Can you work these out from the model? Positions are in its coordinate system, mm. A direction names the side the tool comes from. Round coordinates to 2 decimals unless told otherwise and drop trailing zeros. Loops run counter-clockwise (first coordinate to the right, second up) from the corner with the lowest first, then second, coordinate; pieces in that order, holes last. Notation, with made-up numbers: M -26.75,38 L 13.25,38 A26 cw 13.25,69 Z; hole C 4.5,-30.5 d10. An arc over 180 degrees is marked long. Return JSON: item names as keys, results as strings.
```python
from build123d import *

# Parameters (mm, degrees)
SKETCH_2_W          = 60
SKETCH_2_H          = 39
EXTRUDE_1_DEPTH     = 70
SKETCH_3_R          = 50
EXTRUDE_2_DEPTH     = 43
FILLET_1_R          = 5
FILLET_2_R          = 5
SKETCH_4_R          = 1.5
CUT_EXTRUDE_1_DEPTH = 3.5
SKETCH_5_R          = 1.5
CUT_EXTRUDE_2_DEPTH = 3.5


with BuildPart() as part:
    # 草图2 → 凸台-拉伸1 (new body)
    with BuildSketch(Plane(origin=(0, 0, 0), x_dir=(0, 0, -1), z_dir=(1, 0, 0))):
        Rectangle(SKETCH_2_W, SKETCH_2_H)
    extrude(amount=EXTRUDE_1_DEPTH)

    # 草图3 → 凸台-拉伸2 (add)
    with BuildSketch(Plane(origin=(70, 0, 0), x_dir=(0, 0, -1), z_dir=(1, 0, 0))):
        Circle(SKETCH_3_R)
    extrude(amount=-EXTRUDE_2_DEPTH)

    # 圆角1
    fillet_1_edges = [part.edges().sort_by_distance(p)[0] for p in [
        (70, 0, 50),
    ]]
    fillet(fillet_1_edges, radius=FILLET_1_R)

    # 圆角2
    fillet_2_edges = [part.edges().sort_by_distance(p)[0] for p in [
        (27, 0, 50),
    ]]
    fillet(fillet_2_edges, radius=FILLET_2_R)

    # 草图4 → 切除-拉伸1 (cut)
    with BuildSketch(Plane(origin=(0, 19.5, 0), x_dir=(1, 0, 0), z_dir=(0, 1, 0))):
        with Locations(Location((13, 0, 0), (0, 0, 270))):
            Circle(SKETCH_4_R)
    extrude(amount=-CUT_EXTRUDE_1_DEPTH, mode=Mode.SUBTRACT)

    # 草图5 → 切除-拉伸2 (cut)
    with BuildSketch(Plane.XZ.offset(19.5)):
        with Locations(Location((8, 13.5, 0), (0, 0, 270))):
            Circle(SKETCH_5_R)
        with Locations(Location((8, -13.25, 0), (0, 0, 270))):
            Circle(SKETCH_5_R)
    extrude(amount=-CUT_EXTRUDE_2_DEPTH, mode=Mode.SUBTRACT)


solid = part.part
```
Q1. I'm going to push flat-ended pins straight in: pin 1 Ø12 at (x, y) = (43, 26) entering from -Z; pin 2 Ø3 at (x, y) = (40, 4) entering from +Z; pin 3 Ø1 at (x, y) = (33.5, 25.5) entering from -Z. Where does each tip first touch, or does it pass through?
Results:
{"pin 1": "stops at z = -45.83", "pin 2": "stops at z = 49.94", "pin 3": "stops at z = -43.3"}
Q2. If I drill on line 1 along X through (y, z) = (18.35, 0); line 2 along X through (y, z) = (-18.25, 13.5); line 3 along X through (y, z) = (37, 0.5), over which ranges is the centre line in solid material (lowest first)?
Results:
{"line 1": "x = 0 to 11.5, 14.5 to 70", "line 2": "x = 0 to 6.5, 9.5 to 70", "line 3": "x = 27 to 70"}
Q3. Suppose I cut it at A-A, the plane y = 0. Please give me the cut outline in (x, z), plus the area to 3 significant figures.
Results:
{"outline": "M 0,-30 L 27,-30 L 27,-45 A5 ccw 32,-50 L 65,-50 A5 ccw 70,-45 L 70,45 A5 ccw 65,50 L 32,50 A5 ccw 27,45 L 27,30 L 0,30 Z", "area": "5,900 mm2"}
Q4. Suppose I cut it at C-C, the plane z = 0. Please give me the cut outline in (x, y), plus the area to 3 significant figures.
Results:
{"outline": "M 0,-19.5 L 27,-19.5 L 27,-45 A5 ccw 32,-50 L 65,-50 A5 ccw 70,-45 L 70,45 A5 ccw 65,50 L 32,50 A5 ccw 27,45 L 27,19.5 L 14.5,19.5 L 14.5,16 L 11.5,16 L 11.5,19.5 L 0,19.5 Z", "area": "5,320 mm2"}
Q5. On a 3-axis mill with a long thin cutter (end or side, diameter ignored), from which of +Z, -Z, +X, -X, +Y, -Y can I reach the whole of each face in a straight line? I mean faces 4 (the cylindrical face through (13.45, 17.77, 1.43)), 5 (the flat face through (13, -19.5, 0)), 6 (the flat face through (16, 19.5, 0)). Say none if no direction works.
Results:
{"face 4": "+Y", "face 5": "+Z, -Z, -X, -Y", "face 6": "+Z, -Z, -X, +Y"}
Q6. Suppose I cut it at D-D, the plane x = 36.5. Please give me the cut outline in (y, z).
Results:
{"outline": "C 0,0 d100"}
Q7. Thinking about a two-plate mould opening in Z: for faces 1 (the cylindrical face through (7.09, -17.77, -12.06)), 2 (the cylindrical face through (48.73, 15.02, -47.69)), 3 (the flat face through (13, 0, -30)), which applies, pulls with the +Z half, pulls with the -Z half, needs draft (parallel to the pull), parting line crosses it, or undercut?
Results:
{"face 1": "undercut", "face 2": "parting line crosses it", "face 3": "pulls with the -Z half"}
Q8. Suppose I cut it at B-B, the plane x = 8. Please give me the cut outline in (y, z), plus the area to 3 significant figures.
Results:
{"outline": "M -19.5,-30 L 19.5,-30 L 19.5,30 L -19.5,30 L -19.5,15 L -16,15 L -16,12 L -19.5,12 L -19.5,-11.75 L -16,-11.75 L -16,-14.75 L -19.5,-14.75 Z", "area": "2,320 mm2"}
